```python
from build123d import *

# Parameters (mm, degrees)
SKETCH1_W                                       = 317.5
SKETCH1_H                                       = 50.8
BOSS_EXTRUDE1_DEPTH                             = 6.35
CBORE_FOR_10_SOCKET_HEAD_CAP_SCREW1_D           = 5.1054
CBORE_FOR_10_SOCKET_HEAD_CAP_SCREW1_CBORE_D     = 9.525
CBORE_FOR_10_SOCKET_HEAD_CAP_SCREW1_CBORE_DEPTH = 4.826
F_1_4_0_25_DIAMETER_HOLE1_D                     = 6.35
F_6_32_TAPPED_HOLE1_D                           = 2.7051
SKETCH12_W                                      = 31.75
SKETCH12_H                                      = 25.4
BOSS_EXTRUDE3_DEPTH                             = 6.35
F_1_4_0_25_DIAMETER_HOLE2_D                     = 6.35


with BuildPart() as part:
    # Sketch1 → Boss-Extrude1 (new body)
    with BuildSketch(Plane(origin=(0, 0, 0), x_dir=(1, 0, 0), z_dir=(0, 1, 0))):
        Rectangle(SKETCH1_W, SKETCH1_H)
    extrude(amount=BOSS_EXTRUDE1_DEPTH)

    # CBORE for #10 Socket Head Cap Screw1 (through all)
    with Locations(Plane(origin=(0, 6.35, 0), x_dir=(1, 0, 0), z_dir=(0, 1, 0))):
        with Locations((-125.73, -12.7), (19.05, 12.7), (69.85, 12.7), (19.05, -12.7), (69.85, -12.7), (-125.73, 12.7), (-125.73, 0)):
            CounterBoreHole(CBORE_FOR_10_SOCKET_HEAD_CAP_SCREW1_D / 2, CBORE_FOR_10_SOCKET_HEAD_CAP_SCREW1_CBORE_D / 2, CBORE_FOR_10_SOCKET_HEAD_CAP_SCREW1_CBORE_DEPTH)

    # 1/4 (0.25) Diameter Hole1 (through all)
    with Locations(Plane.XZ):
        with Locations((-146.05, 12.7), (-146.05, 0), (-146.05, -12.7), (146.05, 12.7), (146.05, 0), (146.05, -12.7)):
            Hole(F_1_4_0_25_DIAMETER_HOLE1_D / 2)

    # #6-32 Tapped Hole1 (through all)
    with Locations(Plane(origin=(0, 0, 0), x_dir=(-1, 0, 0), z_dir=(0, -1, 0))):
        with Locations((57.15, 0)):
            Hole(F_6_32_TAPPED_HOLE1_D / 2)

    # Sketch12 → Boss-Extrude3 (add)
    with BuildSketch(Plane(origin=(0, 6.35, 0), x_dir=(1, 0, 0), z_dir=(0, 1, 0))):
        with Locations((-57.15, -38.1)):
            Rectangle(SKETCH12_W, SKETCH12_H)
    extrude(amount=-BOSS_EXTRUDE3_DEPTH)

    # 1/4 (0.25) Diameter Hole2 (through all)
    with Locations(Plane(origin=(0, 0, 0), x_dir=(-1, 0, 0), z_dir=(0, -1, 0))):
        with Locations((52.07, -43.18), (62.23, -33.02)):
            Hole(F_1_4_0_25_DIAMETER_HOLE2_D / 2)


solid = part.part
```
Input: part model. Units: mm. Frame: model coordinates. A direction names the side the tool comes from. Give positions to 0.01 mm unless a question says otherwise; leave off trailing zeros. Order: outer loops, then holes, each group sorted by start corner. A loop starts at its lowest first (then second) coordinate and runs counter-clockwise, first axis right, second up. Notation, with made-up numbers: M -27,-35 L 18,-35 A23 ccw 18,-27 Z; hole C 60.5,78 d6. An arc over 180 degrees is marked long. One line per question, with ' | ' between items.
1) Section B-B on x = -62.23. Output: boundary loops of the cut face in (y, z) (3 decimals).
Filled in:
outline: M 0,-25.4 L 6.35,-25.4 L 6.35,29.845 L 0,29.845 Z; M 0,36.195 L 6.35,36.195 L 6.35,50.8 L 0,50.8 Z
2) Access query for faces 1 (the face through (67.5, 0.8, 13.7)), 2 (the face through (14.292, 3.971, -12.909)), 3 (the face through (-41.275, 3, 38)). Directions: +Z, -Z, +X, -X, +Y, -Y. A direction counts if a zero-diameter tool reaches every point of the face in a straight line with its end or side. Return the directions, or none.
Filled in:
face 1: +Y, -Y | face 2: +Y | face 3: +Z, +X, +Y, -Y
3) Section C-C on y = 3. State how many separate pieces and enclosed holes the cut face has, and give its area (3 significant figures).
Filled in:
separate pieces: 1 | enclosed holes: 16 | area: 16,200 mm2
4) Contact query for flat-ended pins moving along their axis: P1, Ø7.5, axis at x = -62.23, z = 33.02, coming from the +Y side; P2, Ø5, axis at x = 21, z = -12.5, coming from the +Y side; P3, Ø1.5, axis at x = 39.5, y = 5, coming from the +Z side; P4, Ø3, axis at y = 4.5, z = 43, coming from the +X side (3 decimals). Output: stop coordinate, or through.
Filled in:
P1: stops at y = 6.35 | P2: stops at y = 1.52 | P3: stops at z = 25.4 | P4: stops at x = -41.275
5) Section A-A on z = 33.02. Output: boundary loops of the cut face in (x, y) (3 decimals), and give its area (3 significant figures).
Filled in:
outline: M -73.025,0 L -65.405,0 L -65.405,6.35 L -73.025,6.35 Z; M -59.055,0 L -41.275,0 L -41.275,6.35 L -59.055,6.35 Z | area: 161 mm2
6) Section D-D on x = -146.05. Output: boundary loops of the cut face in (y, z) (3 decimals), and give its area (3 significant figures).
Filled in:
outline: M 0,-25.4 L 6.35,-25.4 L 6.35,-15.875 L 0,-15.875 Z; M 0,-9.525 L 6.35,-9.525 L 6.35,-3.175 L 0,-3.175 Z; M 0,3.175 L 6.35,3.175 L 6.35,9.525 L 0,9.525 Z; M 0,15.875 L 6.35,15.875 L 6.35,25.4 L 0,25.4 Z | area: 202 mm2
7) Draft query along Z for faces 4 (the face through (72.41, 3.971, 8.684)), 5 (the face through (57, 3, 25.4)), 6 (the face through (-73.025, 3, 38)). Return one class per face: pulls with the +Z half, pulls with the -Z half, needs draft (parallel to the pull), parting line crosses it, or undercut.
Filled in:
face 4: undercut | face 5: pulls with the +Z half | face 6: needs draft
8) Ray query, L1, parallel to X at y = 4, z = 13; L2, parallel to Z at x = 19.05, y = 5.3; L3, parallel to Z at x = -125.73, y = 0.8. Return the intervals inside material, ascending.
Filled in:
L1: x = -158.75 to -149.21, -142.89 to -130.48, -120.98 to 14.3, 23.8 to 65.1, 74.6 to 142.89, 149.21 to 158.75 | L2: z = -25.4 to -17.46, -7.94 to 7.94, 17.46 to 25.4 | L3: z = -25.4 to -15.25, -10.15 to -2.55, 2.55 to 10.15, 15.25 to 25.4
